Source: CAD feature listing. Evaluate the final solid. Frame: model axes, mm. Face numbers are marked on the shaded views. A direction names the side the tool comes from. Give positions to 0.01 mm unless a question says otherwise; leave off trailing zeros. Order: outer loops, then holes, each group sorted by start corner. A loop starts at its lowest first (then second) coordinate and runs counter-clockwise, first axis right, second up. Notation, with made-up numbers: (39.5, 87) -> (66.5, 87) arc R30 cw to (66.5, 109) -> close; hole circle Ø10 at (43.5, 84). An arc over 180 degrees is marked (long way). Use CSV: the item, a comma, the result in double quotes.
Autodesk Inventor part; units mm, degrees
ref_plane "Work Plane1" through (0, 15, 0) normal (0, 1, 0) x (-1, 0, 0)
ref_plane "YZ Plane" through (0, 0, 0) normal (1, 0, 0) x (0, 1, 0)
ref_plane "XY Plane" through (0, 0, 0) normal (0, 0, 1) x (1, 0, 0)
sketch "Sketch1" plane through (0, 0, 0) normal (0, 0, 1) x (1, 0, 0)
  line L0 (0, 0) -> (0, 15)
  line L1 (0, 0) -> (15, 0)
  arc A0 (15, 0) -> (0, 15) centre (0, 0) ccw
  line L2 (0, -3.621321) -> (0, 21.727922)
  dimension "d2" = 15
sketch "Sketch1 outline for Revolution1" plane through (0, 0, 0) normal (0, 0, 1) x (1, 0, 0)
  line L0 (0, 0) -> (0, 15)
  arc A0 (0, 15) -> (15, 0) centre (0, 0) cw
  line L1 (15, 0) -> (0, 0)
revolve "Revolution1" add sketch "Sketch1 outline for Revolution1" angle 360 about axis through (0, -10, 0) along (0, 1, 0)
ref_plane "Work Plane1" through (0, 15, 0) normal (0, 1, 0) x (-1, 0, 0)
sketch "Sketch2" plane through (0, 15, 0) normal (0, 1, 0) x (-1, 0, 0)
  point P0 (0, 0)
  point P1 (0, 0)
hole "Hole1" at (0, 15, 0) direction (0, -1, 0) diameter 4.5 end through all counterbore diameter 8 counterbore depth 4
shell "Shell1" thickness 3 removed faces 1 at (10.599241, 0, 1.286981)
sketch "Sketch3" plane through (0, 0, 0) normal (0, -1, 0) x (1, 0, 0)
  circle A0 centre (0, 0) radius 5.25
  circle A1 centre (0, 0) radius 2.25
sketch "Sketch3 outline for Extrusion1" plane through (0, 0, 0) normal (0, -1, 0) x (1, 0, 0)
  circle A0 centre (0, 0) radius 5.25
  circle A1 centre (0, 0) radius 2.25
extrude "Extrusion1" cut sketch "Sketch3 outline for Extrusion1" against normal blind 8
properties part number "Ball_Upper Half" material "Nylon 6/6"
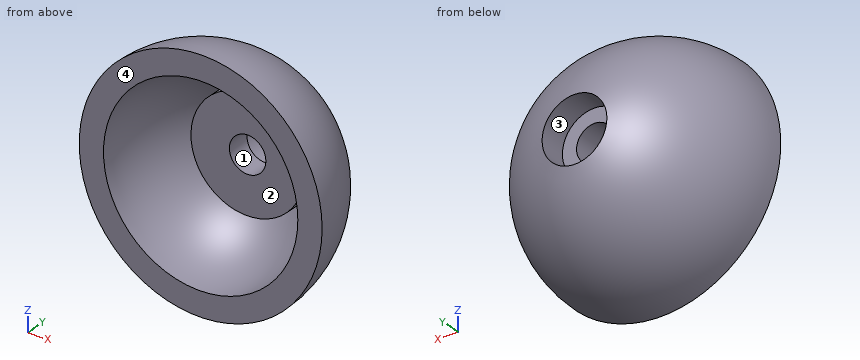
1. Section query A-A on z = 0. Return loops of the section in (x, y).
Answer below:
outline,"(-15, 0) -> (-12, 0) arc R12 cw to (-7, 9.75) -> (-7, 8) -> (-2.25, 8) -> (-2.25, 11) -> (-4, 11) -> (-4, 14.46) arc R15 ccw to start; (2.25, 8) -> (7, 8) -> (7, 9.75) arc R12 cw to (12, 0) -> (15, 0) arc R15 ccw to (4, 14.46) -> (4, 11) -> (2.25, 11) -> close"
2. Section query D-D on z = 5.5. Return loops of the section in (x, y).
Answer below:
outline,"(-13.96, 0) -> (-10.67, 0) arc R10.67 cw to (-4.33, 9.75) -> (-4.33, 8) -> (4.33, 8) -> (4.33, 9.75) arc R10.67 cw to (10.67, 0) -> (13.96, 0) arc R13.96 ccw to start"
3. Pin query (flat end, axial travel): P1, Ø7, axis at x = 0, z = 0, coming from the +Y side; P2, Ø2, axis at y = 11, z = -3.5, coming from the -X side; P3, Ø1, axis at x = -8, y = 8, coming from the -Z side. Return the tip coordinate at first contact, or that it passes through.
Answer below:
P1,"stops at y = 11"
P2,"stops at x = -10.67"
P3,"stops at z = -10.4"
4. Section query C-C on x = 6.25. Return loops of the section in (y, z), plus the area to 3 significant figures.
Answer below:
outline,"(0, -13.64) arc R13.64 ccw to (0, 13.64) -> (0, 10.24) arc R10.24 cw to (9.75, 3.15) -> (8, 3.15) -> (8, -3.15) -> (9.75, -3.15) arc R10.24 cw to (0, -10.24) -> close"
area,"140 mm²"
5. Ray query, line 1 along X through (y, z) = (13, 0); line 2 along X through (y, z) = (2.75, -6.75); line 3 along Y through (x, z) = (-2.75, 0.25). Return the intervals inside material, ascending.
Answer below:
line 1,"x = -7.48 to -4, 4 to 7.48"
line 2,"x = -13.11 to -9.53, 9.53 to 13.11"
line 3,"y = 8 to 11"
6. Section query B-B on x = -1.75. Return loops of the section in (y, z), plus the area to 3 significant figures.
Answer below:
outline,"(0, -14.9) arc R14.9 ccw to (14.46, -3.6) -> (11, -3.6) -> (11, -1.41) -> (8, -1.41) -> (8, -6.78) -> (9.75, -6.78) arc R11.87 cw to (0, -11.87) -> close; (0, 11.87) arc R11.87 cw to (9.75, 6.78) -> (8, 6.78) -> (8, 1.41) -> (11, 1.41) -> (11, 3.6) -> (14.46, 3.6) arc R14.9 ccw to (0, 14.9) -> close"
area,"135 mm²"
7. Mould query, pull axis X, two halves, no side actions, for the marked faces 3 and 4. Classes: released by +X, released by -X, zero draft, split by the parting line, or undercut.
Answer below:
face 3,"undercut"
face 4,"zero draft"
8. Access query for the marked faces 1 and 2. Directions: +Z, -Z, +X, -X, +Y, -Y. A direction counts if a zero-diameter tool reaches every point of the face in a straight line with its end or side. Return the directions, or none.
Answer below:
face 1,"+Y, -Y"
face 2,"-Y"
